Could you check a few things on this drawing? It's one solid part, dimensions in mm from its lowest x, y, z. Give positions to 0.01 mm unless a question says otherwise; leave off trailing zeros. Write each loop counter-clockwise with the first axis right and the second up, starting at its lowest first coordinate (ties: lowest second). Pieces come first, ordered by that corner, then holes. Notation, with made-up numbers: M 63,74.25 L 87,74.25 A24 ccw 87,113.25 Z; hole C 56,82.5 d9. An arc over 180 degrees is marked long. Answer as CSV lines item,"result". Start each with the question number.
Q1. Suppose I cut it at A-A (x = 49.5). Write out the boundary of the cut face in (y, z), then the cut area to 3 significant figures.
Q2. Thinking about a two-plate mould opening in X: for the marked faces 1, 2 and 3, which applies, +X half, -X half, draft (parallel to the pull), parting line (faces both ways), or undercut?
Q3. For pin 1 (4 mm diameter, centred on y = 4.5, z = 47, fed in from +X); pin 2 (6 mm diameter, centred on y = 2.5, z = 38, fed in from -X); pin 3 (6 mm diameter, centred on x = 27.5, z = 5.5, fed in from +Y), each with a flat end and sliding along its axis, tell me the tip position at first contact or that it passes through.
Q4. Suppose I cut it at B-B (z = 27.5). Write out the boundary of the cut face in (x, y), then the cut area to 4 significant figures.
Q5. Suppose I cut it at D-D (y = 1.75). Write out the boundary of the cut face in (x, z).
Q6. If I drill on line 1 along X through (y, z) = (1.05, 27.5); line 2 along X through (y, z) = (5.5, 27.5); line 3 along X through (y, z) = (0.95, 49.5), over which ranges is the centre line in solid material (lowest first)?
Q7. Suppose I cut it at C-C (z = 5.5). Write out the boundary of the cut face in (x, y), then the cut area to 3 significant figures.
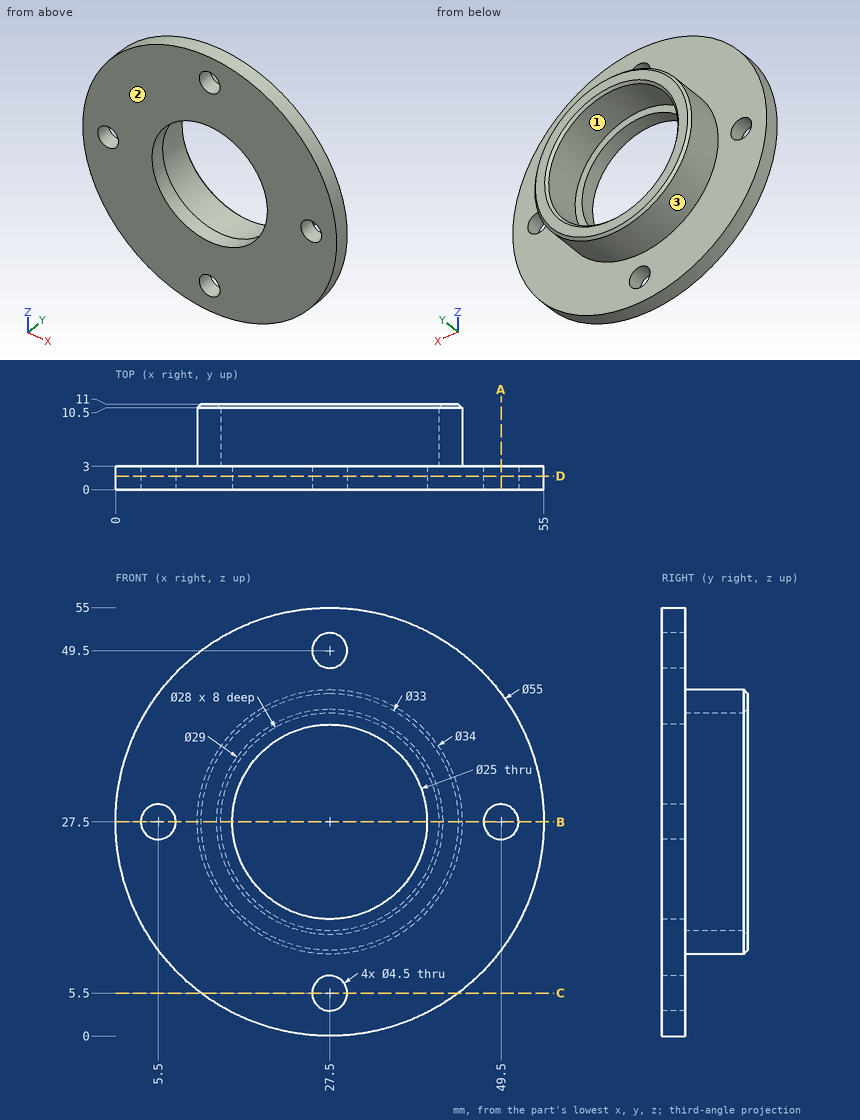
Resolved:
1,outline,"M 0,11 L 3,11 L 3,25.25 L 0,25.25 Z; M 0,29.75 L 3,29.75 L 3,44 L 0,44 Z"
1,area,"85.5 mm^2"
2,face 1,"undercut"
2,face 2,"draft"
2,face 3,"parting line"
3,pin 1,"x = 48.14"
3,pin 2,"x = 1.04"
3,pin 3,"y = 3"
4,outline,"M 0,0 L 3.25,0 L 3.25,3 L 0,3 Z; M 7.75,0 L 15,0 L 15,3 L 13.5,3 L 13.5,10.5 L 13,11 L 11,11 L 10.5,10.5 L 10.5,3 L 7.75,3 Z; M 40,0 L 47.25,0 L 47.25,3 L 44.5,3 L 44.5,10.5 L 44,11 L 42,11 L 41.5,10.5 L 41.5,3 L 40,3 Z; M 51.75,0 L 55,0 L 55,3 L 51.75,3 Z"
4,area,"110.5 mm^2"
5,outline,"C 27.5,27.5 d55; hole C 5.5,27.5 d4.5; hole C 27.5,27.5 d25; hole C 27.5,5.5 d4.5; hole C 27.5,49.5 d4.5; hole C 49.5,27.5 d4.5"
6,line 1,"0 to 3.25, 7.75 to 15, 40 to 47.25, 51.75 to 55"
6,line 2,"10.5 to 13.5, 41.5 to 44.5"
6,line 3,"11 to 25.25, 29.75 to 44"
7,outline,"M 11,0 L 25.25,0 L 25.25,3 L 11,3 Z; M 29.75,0 L 44,0 L 44,3 L 29.75,3 Z"
7,area,"85.5 mm^2"
